Input: part model. Units: mm. Frame: model coordinates. Face numbers are marked on the shaded views. A direction names the side the tool comes from. Give positions to 0.01 mm unless a question says otherwise; leave off trailing zeros. Loops run counter-clockwise (first coordinate to the right, second up) from the corner with the lowest first, then second, coordinate; pieces in that order, holes last. Notation, with made-up numbers: (-14, -13) -> (22, -13) arc R16 ccw to (22, -8) -> close; hole circle Ø6 at (-37, 55.5). An arc over 180 degrees is marked (long way). Answer in a Markdown table with one row per item. Add a question column.
```python
from build123d import *

# Parameters (mm, degrees)
SKETCH1_W           = 4.7625
SKETCH1_H           = 50
SKETCH1_W_2         = 28.575
BOSS_EXTRUDE1_DEPTH = 4.7625
SKETCH1_3_W         = 4.7625
SKETCH1_3_H         = 50
BOSS_EXTRUDE2_DEPTH = 31.75
SKETCH3_W           = 9.525
SKETCH3_H           = 11.1125
SKETCH3_R           = 4
CUT_EXTRUDE1_DEPTH  = 39.1
FILLET1_R           = 6.35


with BuildPart() as part:
    # Sketch1 → Boss-Extrude1 (new body)
    with BuildSketch(Plane(origin=(0, 0, 0), x_dir=(1, 0, 0), z_dir=(0, 1, 0))):
        with Locations((-16.66875, 0)):
            Rectangle(SKETCH1_W, SKETCH1_H)
        Rectangle(SKETCH1_W_2, SKETCH1_H)
        with Locations((16.66875, 0)):
            Rectangle(SKETCH1_W, SKETCH1_H)
    extrude(amount=BOSS_EXTRUDE1_DEPTH)

    # Sketch1<3> → Boss-Extrude2 (add)
    with BuildSketch(Plane(origin=(0, 0, 0), x_dir=(1, 0, 0), z_dir=(0, 1, 0))):
        with Locations((-16.66875, 0)):
            Rectangle(SKETCH1_3_W, SKETCH1_3_H)
        with Locations((16.66875, 0)):
            Rectangle(SKETCH1_3_W, SKETCH1_3_H)
    extrude(amount=-BOSS_EXTRUDE2_DEPTH)

    # Sketch3 → Cut-Extrude1 (cut, through all)
    with BuildSketch(Plane(origin=(19.05, 0, 0), x_dir=(0, 0, -1), z_dir=(1, 0, 0))):
        with Locations((-20.2375, -0.79375)):
            Rectangle(SKETCH3_W, SKETCH3_H)
        with Locations((-16.745, -20.6375)):
            Circle(SKETCH3_R)
    extrude(amount=-CUT_EXTRUDE1_DEPTH, mode=Mode.SUBTRACT)

    # Fillet1
    fillet1_edges = [part.edges().sort_by_distance(p)[0] for p in [
        (-16.66875, -31.75, 25),
        (16.66875, -31.75, 25),
        (-16.66875, -31.75, -25),
        (16.66875, -31.75, -25),
        (-16.66875, -6.35, 15.475),
        (16.66875, -6.35, 15.475),
    ]]
    fillet(fillet1_edges, radius=FILLET1_R)


solid = part.part
```
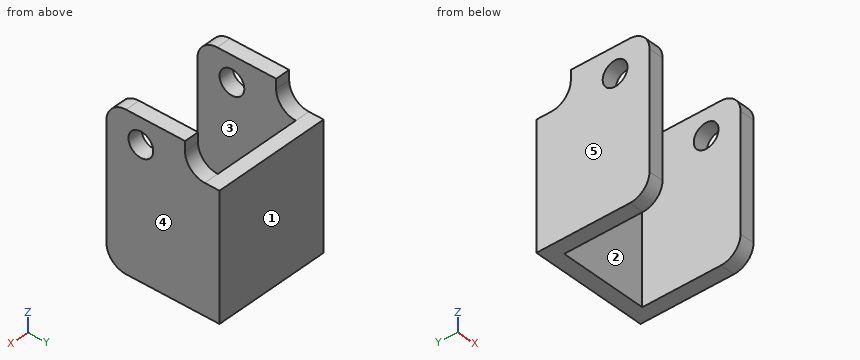
1) Pull-direction query (X, two-part tool) for the marked faces 3, 4 and 5; classes: +X half, -X half, draft (parallel to the pull), parting line (faces both ways), or undercut.
2) Material intervals for line 1 along X through (y, z) = (-17.5, -1); line 2 along Y through (x, z) = (-3, -11), sorted ascending.
3) Reachability of the marked faces 1 and 2 from +Z, -Z, +X, -X, +Y, -Y: full face, straight path, thin tool, end or side. Return the list, or none.
4) Pin query (flat end, axial travel): pin 1 (13 mm diameter, centred on y = -20.64, z = 16.74, fed in from -X); pin 2 (10 mm diameter, centred on x = -8.5, z = 17.5, fed in from -Y); pin 3 (2.5 mm diameter, centred on x = -5.5, y = 2.5, fed in from +Z) (3 decimals); pin 4 (3.5 mm diameter, centred on x = 17.5, z = 24, fed in from +Y). Return the tip coordinate at first contact, or that it passes through.
5) Section A-A on y = -13.5. Output: boundary loops of the cut face in (x, z).
6) Section B-B on z = 20. Output: boundary loops of the cut face in (x, y).
7) Section D-D on z = 7. Output: boundary loops of the cut face in (x, y).
Working result:
| question | item | result |
|---|---|---|
| 1 | face 3 | undercut |
| 1 | face 4 | +X half |
| 1 | face 5 | -X half |
| 2 | line 1 | x = -19.05 to -14.29, 14.29 to 19.05 |
| 2 | line 2 | y = 0 to 4.76 |
| 3 | face 1 | +Z, -Z, +X, -X, +Y |
| 3 | face 2 | +Z, -Z, -Y |
| 4 | pin 1 | stops at x = -19.05 |
| 4 | pin 2 | stops at y = 0 |
| 4 | pin 3 | stops at z = 15.475 |
| 4 | pin 4 | stops at y = -6.35 |
| 5 | outline | (-19.05, -25) -> (-14.29, -25) -> (-14.29, 25) -> (-19.05, 25) -> close; (14.29, -25) -> (19.05, -25) -> (19.05, 25) -> (14.29, 25) -> close |
| 6 | outline | (-19.05, -31.6) -> (-14.29, -31.6) -> (-14.29, -22.96) -> (-19.05, -22.96) -> close; (-19.05, -18.31) -> (-14.29, -18.31) -> (-14.29, -6.08) -> (-19.05, -6.08) -> close; (14.29, -31.6) -> (19.05, -31.6) -> (19.05, -22.96) -> (14.29, -22.96) -> close; (14.29, -18.31) -> (19.05, -18.31) -> (19.05, -6.08) -> (14.29, -6.08) -> close |
| 7 | outline | (-19.05, -31.75) -> (-14.29, -31.75) -> (-14.29, 0) -> (14.29, 0) -> (14.29, -31.75) -> (19.05, -31.75) -> (19.05, 4.76) -> (-19.05, 4.76) -> close |
